Part model, mm, in its own coordinate system. Round coordinates to 2 decimals unless told otherwise and drop trailing zeros. Order: outer loops, then holes, each group sorted by start corner. A loop starts at its lowest first (then second) coordinate and runs counter-clockwise, first axis right, second up. Notation, with made-up numbers: (74, 76.5) -> (93, 76.5) arc R15 cw to (93, 98.5) -> close; hole circle Ø3 at (21, 59). An arc over 180 degrees is marked (long way). Use CSV: the item, a comma, the result in double quotes.
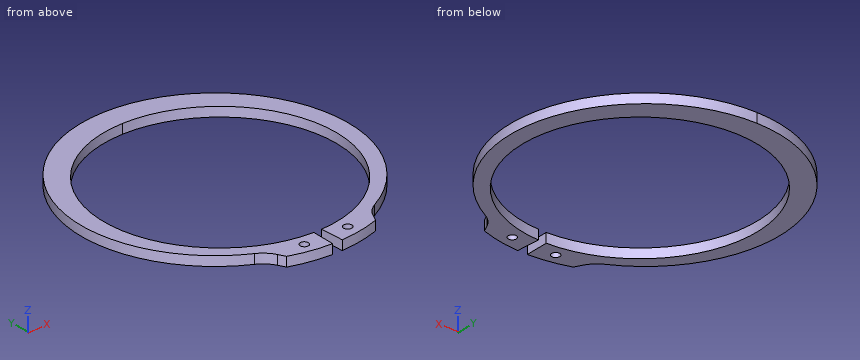
```python
from build123d import *

# Parameters (mm, degrees)
SKETCH4_R           = 1.75
BOSS_EXTRUDE1_DEPTH = 2
FILLET1_R           = 12.038964726


with BuildPart() as part:
    # Sketch4 → Boss-Extrude1 (new, symmetric)
    with BuildSketch(Plane.XY):
        with BuildLine():
            Line((-19.20029003, -55.720637345), (-22.533190866, -49.018953573))
            ThreePointArc((-22.533190866, -49.018953573), (-55.123146751, 14.097654643), (0, 58.9))
            Line((0, 58.9), (0, 49))
            ThreePointArc((0, 49), (-48.992537063, 0.855167915), (-1.710075338, -48.970150524))
            Line((-1.710075338, -48.970150524), (-2.056833323, -58.9))
            ThreePointArc((-2.056833323, -58.9), (-10.746786033, -57.947796794), (-19.20029003, -55.720637345))
        make_face()
        with Locations((-9.371436357, -53.148056637)):
            Circle(SKETCH4_R, mode=Mode.SUBTRACT)
    extrude(amount=BOSS_EXTRUDE1_DEPTH, both=True)

    # Fillet1
    fillet1_edges = [part.edges().sort_by_distance(p)[0] for p in [
        (-22.533190866, -49.018953573, 0),
    ]]
    fillet(fillet1_edges, radius=FILLET1_R)

    # Mirror1: part across plane


with BuildPart() as part_1:
    add(part.part)
    add(part.part.mirror(Plane(origin=(0, 58.9, 2), x_dir=(0, 0, 1), z_dir=(-1, 0, 0))))


solid = part_1.part
```
(1) Cut at A-A, the plane y = -40. Give the cut face in (x, z).
Reply:
outline,"(-36.84, -2) -> (-28.3, -2) -> (-28.3, 2) -> (-36.84, 2) -> close; (28.3, -2) -> (36.84, -2) -> (36.84, 2) -> (28.3, 2) -> close"
(2) Cut at C-C, the plane z = 0.1. Give the cut face in (x, y), then the cut area to 3 significant figures.
Reply:
outline,"(-25.93, -47.4) arc R12.04 cw to (-20.69, -52.73) -> (-19.2, -55.72) arc R58.94 ccw to (-2.06, -58.9) -> (-1.71, -48.97) arc R49 cw (long way) to (1.71, -48.97) -> (2.06, -58.9) arc R58.94 ccw to (19.2, -55.72) -> (20.69, -52.73) arc R12.04 cw to (25.93, -47.4) arc R56.31 ccw (long way) to start; hole circle Ø3.5 at (-9.37, -53.15); hole circle Ø3.5 at (9.37, -53.15)"
area,"2,590 mm2"
(3) Probe probe 1 along Y at (x, z) = (-10.5, -0.4); probe 2 along X at (y, z) = (1.5, -1.8); probe 3 along Y at (x, z) = (5, 0.05). List the from-to ranges inside material, lowest first. Write a range as [from, to].
Reply:
probe 1,"[-57.99, -54.49], [-51.81, -47.86], [47.86, 57.91]"
probe 2,"[-56.3, -48.98], [48.98, 56.3]"
probe 3,"[-58.72, -48.74], [48.74, 58.68]"
(4) Drop a flat-ended pin along its axis: P1, Ø1, axis at x = 7, z = -0.5, coming from the -Y side. Give the stop position or say it passes through.
Reply:
P1,"y = -58.58"
(5) Cut at B-B, the plane x = 35. Give the cut face in (y, z), then the cut area to 3 significant figures.
Reply:
outline,"(-41.53, -2) -> (-34.29, -2) -> (-34.29, 2) -> (-41.53, 2) -> close; (34.29, -2) -> (46.7, -2) -> (46.7, 2) -> (34.29, 2) -> close"
area,"78.6 mm2"
